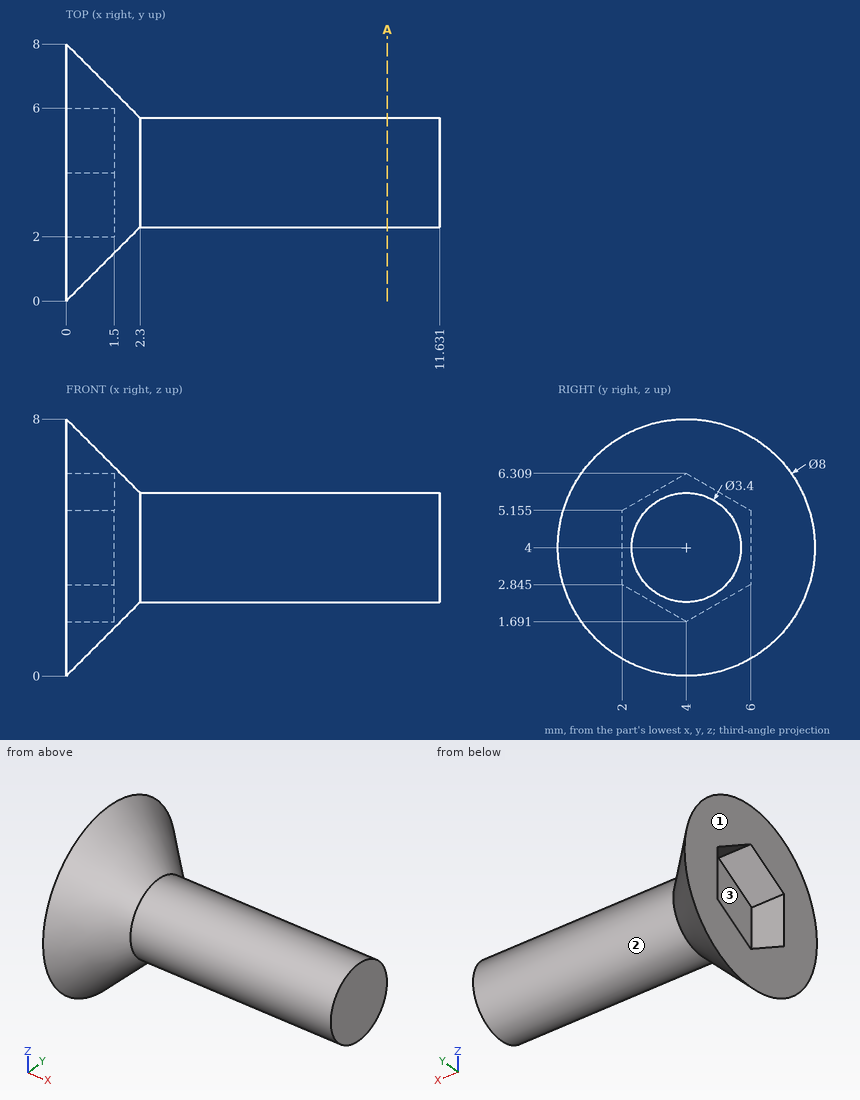
Could you check a few things on this drawing? It's one solid part, dimensions in mm from its lowest x, y, z. A direction names the side the tool comes from. Coordinates: 2 decimals unless noted, no trailing zeros. Order: outer loops, then holes, each group sorted by start corner. A loop starts at its lowest first (then second) coordinate and runs counter-clockwise, first axis right, second up.
1) Imagine slicing it at A-A on x = 10. List the corners of the cut face in (y, z) for me.
2) Which directions (+Z, -Z, +X, -X, +Y, -Y) give clear straight access to the entire face, cutting with the end or side of a thin tool? Please do the marked faces 1, 2 and 3.
3) I need wall thicknesses on line 1 (Z direction, x = 8, y = 5.25); line 2 (X direction, y = 4.5, z = 5.25). Which ranges of each line are inside material? Lowest first, please.
4) Will these pins go through, and if not, where does the flat tip stop? pin 1 (4 mm diameter, centred on x = 7.5, y = 1.5, fed in from +Z) (1 decimal); pin 2 (1.6 mm diameter, centred on x = 0.5, z = 4, fed in from +Y); pin 3 (1.2 mm diameter, centred on x = 0.5, z = 4.5, fed in from -Y); pin 4 (1 mm diameter, centred on x = 2.5, y = 4.5, fed in from -Z).
Response values:
1. outline: circle Ø3.4 at (4, 4)
2. face 1: +Z, -Z, -X, +Y, -Y
2. face 2: +X
2. face 3: -X
3. line 1: z = 2.85 to 5.15
3. line 2: x = 1.5 to 11.63
4. pin 1: stops at z = 5.6
4. pin 2: stops at y = 8
4. pin 3: stops at y = 0
4. pin 4: stops at z = 2.05
